Could you check a few things on this model? Use its own coordinates, in mm. A direction names the side the tool comes from. Coordinates: 2 decimals unless noted, no trailing zeros. Loops run counter-clockwise (first coordinate to the right, second up) from the corner with the lowest first, then second, coordinate; pieces in that order, holes last. Notation, with made-up numbers: (-21.75, 35) -> (23.25, 35) arc R10 cw to (23.25, 42) -> close; hole circle Ø3 at (-14, 36.25). An arc over 180 degrees is marked (long way). One line per question, with ' | ' between items.
from build123d import *
from OCP.BRepFilletAPI import BRepFilletAPI_MakeChamfer
from build123d.topology import SkipClean

# Parameters (mm, degrees)
SZKIC2_R                         = 1.25
DODANIE_WYCI_GNI_CIE2_DEPTH      = 2
DODANIE_WYCI_GNI_CIE3_DEPTH      = 3
DODANIE_WYCI_GNI_CIE3_DEPTH_BACK = 2
SZKIC3_W                         = 6
SZKIC3_H                         = 30
DODANIE_WYCI_GNI_CIE4_DEPTH      = 30
DODANIE_WYCI_GNI_CIE4_DEPTH_BACK = 2
SZKIC4_W                         = 6
SZKIC4_H                         = 3
SFAZOWANIE1_SIZE                 = 8
SFAZOWANIE1_SIZE2                = 7.929766182
SFAZOWANIE1_SIZE2_2              = 8.072133677
SFAZOWANIE2_SIZE                 = 10
SFAZOWANIE3_SIZE                 = 3
SZKIC5_W                         = 38.5
SZKIC5_H                         = 53.3
SZKIC5_W_2                       = 38.438336307
SZKIC5_H_2                       = 53.191798748
WYTNIJ_WYCI_GNI_CIE1_DEPTH       = 48.5
DODANIE_WYCI_GNI_CIE5_DEPTH      = 42.061663693
WYTNIJ_WYCI_GNI_CIE2_DEPTH       = 50.5


with BuildPart() as part:
    # Szkic2 → Dodanie-wyciągnięcie2 (new body)
    with BuildSketch(Plane.XY):
        with BuildLine():
            Line((-191.460111356, 62.995312244), (-303.460111356, 62.995312244))
            Line((-303.460111356, 62.995312244), (-308.460111356, 57.995312244))
            Line((-308.460111356, 57.995312244), (-308.460111356, 23.495312244))
            Line((-308.460111356, 23.495312244), (-303.460111356, 18.495312244))
            Line((-303.460111356, 18.495312244), (-302.736783969, 18.495312244))
            ThreePointArc((-302.736783969, 18.495312244), (-304.359873615, 24.570533036), (-302.660111356, 30.624749412))
            Line((-302.660111356, 30.624749412), (-302.660111356, 55.958269629))
            ThreePointArc((-302.660111356, 55.958269629), (-301.800506396, 56.364057485), (-301.339420723, 57.195312244))
            Line((-301.339420723, 57.195312244), (-283.580801989, 57.195312244))
            ThreePointArc((-283.580801989, 57.195312244), (-283.119716316, 56.364057485), (-282.260111356, 55.958269629))
            Line((-282.260111356, 55.958269629), (-282.260111356, 30.624749412))
            ThreePointArc((-282.260111356, 30.624749412), (-280.560349096, 24.570533036), (-282.183438743, 18.495312244))
            Line((-282.183438743, 18.495312244), (-257.736783969, 18.495312244))
            ThreePointArc((-257.736783969, 18.495312244), (-259.359873615, 24.570533036), (-257.660111356, 30.624749412))
            Line((-257.660111356, 30.624749412), (-257.660111356, 55.958269629))
            ThreePointArc((-257.660111356, 55.958269629), (-256.800506396, 56.364057485), (-256.339420723, 57.195312244))
            Line((-256.339420723, 57.195312244), (-238.580801989, 57.195312244))
            ThreePointArc((-238.580801989, 57.195312244), (-238.119716316, 56.364057485), (-237.260111356, 55.958269629))
            Line((-237.260111356, 55.958269629), (-237.260111356, 30.624749412))
            ThreePointArc((-237.260111356, 30.624749412), (-235.561787998, 24.695065265), (-237.060111356, 18.711714747))
            Line((-237.060111356, 18.711714747), (-212.736783969, 18.495312244))
            ThreePointArc((-212.736783969, 18.495312244), (-214.359873615, 24.570533036), (-212.660111356, 30.624749412))
            Line((-212.660111356, 30.624749412), (-212.660111356, 55.958269629))
            ThreePointArc((-212.660111356, 55.958269629), (-211.800506396, 56.364057485), (-211.339420723, 57.195312244))
            Line((-211.339420723, 57.195312244), (-193.580801989, 57.195312244))
            ThreePointArc((-193.580801989, 57.195312244), (-193.119716316, 56.364057485), (-192.260111356, 55.958269629))
            Line((-192.260111356, 55.958269629), (-192.260111356, 30.624749412))
            ThreePointArc((-192.260111356, 30.624749412), (-190.560349096, 24.570533036), (-192.183438743, 18.495312244))
            Line((-192.183438743, 18.495312244), (-191.460111356, 18.495312244))
            Line((-191.460111356, 18.495312244), (-186.460111356, 23.495312244))
            Line((-186.460111356, 23.495312244), (-186.460111356, 57.995312244))
            Line((-186.460111356, 57.995312244), (-191.460111356, 62.995312244))
        make_face()
        with Locations((-305.960111356, 31.245312244)):
            Circle(SZKIC2_R, mode=Mode.SUBTRACT)
        with Locations((-278.960111356, 31.245312244)):
            Circle(SZKIC2_R, mode=Mode.SUBTRACT)
        with Locations((-305.960111356, 39.245312244)):
            Circle(SZKIC2_R, mode=Mode.SUBTRACT)
        with Locations((-278.960111356, 39.245312244)):
            Circle(SZKIC2_R, mode=Mode.SUBTRACT)
        with Locations((-260.960111356, 31.245312244)):
            Circle(SZKIC2_R, mode=Mode.SUBTRACT)
        with Locations((-260.960111356, 39.245312244)):
            Circle(SZKIC2_R, mode=Mode.SUBTRACT)
        with Locations((-233.960111356, 31.245312244)):
            Circle(SZKIC2_R, mode=Mode.SUBTRACT)
        with Locations((-233.960111356, 39.245312244)):
            Circle(SZKIC2_R, mode=Mode.SUBTRACT)
        with Locations((-215.960111356, 31.245312244)):
            Circle(SZKIC2_R, mode=Mode.SUBTRACT)
        with Locations((-188.960111356, 31.245312244)):
            Circle(SZKIC2_R, mode=Mode.SUBTRACT)
        with Locations((-215.960111356, 39.245312244)):
            Circle(SZKIC2_R, mode=Mode.SUBTRACT)
        with Locations((-188.960111356, 39.245312244)):
            Circle(SZKIC2_R, mode=Mode.SUBTRACT)
        with Locations((-305.960111356, 47.245312244)):
            Circle(SZKIC2_R, mode=Mode.SUBTRACT)
        with Locations((-278.960111356, 47.245312244)):
            Circle(SZKIC2_R, mode=Mode.SUBTRACT)
        with Locations((-260.960111356, 47.245312244)):
            Circle(SZKIC2_R, mode=Mode.SUBTRACT)
        with Locations((-305.960111356, 55.245312244)):
            Circle(SZKIC2_R, mode=Mode.SUBTRACT)
        with Locations((-278.960111356, 55.245312244)):
            Circle(SZKIC2_R, mode=Mode.SUBTRACT)
        with Locations((-300.460111356, 60.495312244)):
            Circle(SZKIC2_R, mode=Mode.SUBTRACT)
        with Locations((-284.460111356, 60.495312244)):
            Circle(SZKIC2_R, mode=Mode.SUBTRACT)
        with Locations((-260.960111356, 55.245312244)):
            Circle(SZKIC2_R, mode=Mode.SUBTRACT)
        with Locations((-255.460111356, 60.495312244)):
            Circle(SZKIC2_R, mode=Mode.SUBTRACT)
        with Locations((-233.960111356, 47.245312244)):
            Circle(SZKIC2_R, mode=Mode.SUBTRACT)
        with Locations((-215.960111356, 47.245312244)):
            Circle(SZKIC2_R, mode=Mode.SUBTRACT)
        with Locations((-188.960111356, 47.245312244)):
            Circle(SZKIC2_R, mode=Mode.SUBTRACT)
        with Locations((-233.960111356, 55.245312244)):
            Circle(SZKIC2_R, mode=Mode.SUBTRACT)
        with Locations((-239.460111356, 60.495312244)):
            Circle(SZKIC2_R, mode=Mode.SUBTRACT)
        with Locations((-215.960111356, 55.245312244)):
            Circle(SZKIC2_R, mode=Mode.SUBTRACT)
        with Locations((-188.960111356, 55.245312244)):
            Circle(SZKIC2_R, mode=Mode.SUBTRACT)
        with Locations((-210.460111356, 60.495312244)):
            Circle(SZKIC2_R, mode=Mode.SUBTRACT)
        with Locations((-194.460111356, 60.495312244)):
            Circle(SZKIC2_R, mode=Mode.SUBTRACT)
    extrude(amount=DODANIE_WYCI_GNI_CIE2_DEPTH)

    # Szkic3 → Dodanie-wyciągnięcie3 (add, two sides: drawn at the far end of the back side and taken through both)
    with BuildSketch(Plane.XY.offset(2).offset(-DODANIE_WYCI_GNI_CIE3_DEPTH_BACK)):
        with Locations((-269.960111356, 27.695312244)):
            Rectangle(SZKIC3_W, SZKIC3_H)
        with Locations((-224.898447663, 27.803513496)):
            Rectangle(SZKIC3_W, SZKIC3_H)
    extrude(amount=DODANIE_WYCI_GNI_CIE3_DEPTH + DODANIE_WYCI_GNI_CIE3_DEPTH_BACK)

    # Szkic4 → Dodanie-wyciągnięcie4 (add, two sides: drawn at the far end of the back side and taken through both)
    with BuildSketch(Plane.XY.offset(2).offset(-DODANIE_WYCI_GNI_CIE4_DEPTH_BACK)):
        with Locations((-269.960111356, 11.195312244)):
            Rectangle(SZKIC4_W, SZKIC4_H)
        with Locations((-224.898447663, 11.303513496)):
            Rectangle(SZKIC4_W, SZKIC4_H)
    extrude(amount=DODANIE_WYCI_GNI_CIE4_DEPTH + DODANIE_WYCI_GNI_CIE4_DEPTH_BACK)

    # Sfazowanie1: one chamfer whose edges measure the first distance from different faces: ONE call of the kernel's chamfer builder (chamfer() names one face for all edges)
    sfazowanie1_edges_1 = [part.edges().sort_by_distance(p)[0] for p in [
        (-266.960111356, 18.495312244, 1),
        (-272.960111356, 18.495312244, 1),
    ]]
    sfazowanie1_edges_2 = [part.edges().sort_by_distance(p)[0] for p in [
        (-221.898447663, 18.57682276, 1),
    ]]
    sfazowanie1_side_2 = [part.faces().sort_by_distance(p)[0] for p in [
        (-221.898447663, 14.190168128, 0.459673797),
    ]]
    sfazowanie1_edges_3 = [part.edges().sort_by_distance(p)[0] for p in [
        (-227.898447663, 18.630204232, 1),
    ]]
    sfazowanie1_side_3 = [part.faces().sort_by_distance(p)[0] for p in [
        (-227.898447663, 42.343839698, 3.5),
    ]]
    sfazowanie1 = BRepFilletAPI_MakeChamfer(part.part.solid().wrapped)
    for e in sfazowanie1_edges_1:
        sfazowanie1.Add(SFAZOWANIE1_SIZE, e.wrapped)
    for e in sfazowanie1_edges_2:
        sfazowanie1.Add(SFAZOWANIE1_SIZE, SFAZOWANIE1_SIZE2, e.wrapped, sfazowanie1_side_2[0].wrapped)  # the first distance lies on this face
    for e in sfazowanie1_edges_3:
        sfazowanie1.Add(SFAZOWANIE1_SIZE, SFAZOWANIE1_SIZE2_2, e.wrapped, sfazowanie1_side_3[0].wrapped)  # the first distance lies on this face
    add(Compound.cast(sfazowanie1.Shape()), mode=Mode.REPLACE)

    # Sfazowanie2
    sfazowanie2_edges = [part.edges().sort_by_distance(p)[0] for p in [
        (-269.960111356, 12.695312244, 5),
        (-224.898447663, 12.803513496, 5),
    ]]
    chamfer(sfazowanie2_edges, length=SFAZOWANIE2_SIZE)

    # Sfazowanie3
    sfazowanie3_edges = [part.edges().sort_by_distance(p)[0] for p in [
        (-224.898447663, 12.803513496, 32),
        (-269.960111356, 12.695312244, 32),
        (-224.898447663, 42.803513496, 5),
        (-269.960111356, 42.695312244, 5),
    ]]
    chamfer(sfazowanie3_edges, length=SFAZOWANIE3_SIZE - 0.0001)  # a hair under: the kernel refuses the full size

    # Szkic5 → Wytnij-wyciągnięcie1 (cut, symmetric)
    with BuildSketch(Plane.XY.offset(2)):
        with Locations((-289.210111356, 36.345312244)):
            Rectangle(SZKIC5_W, SZKIC5_H)
        with Locations((-205.67927951, 36.39941287)):
            Rectangle(SZKIC5_W_2, SZKIC5_H_2)
    extrude(amount=WYTNIJ_WYCI_GNI_CIE1_DEPTH, both=True, mode=Mode.SUBTRACT)

    # Szkic6 → Dodanie-wyciągnięcie5 (add)
    with SkipClean():  # the faces are left unmerged after this step: merging them gives an invalid solid
        with BuildSketch(Plane(origin=(-266.960111356, 0, 0), x_dir=(0, 0, -1), z_dir=(1, 0, 0))):
            Polygon((-32, 9.695312244), (-29, 12.695312244), (0, 12.695312244), (0, 9.695312244), align=None)
        extrude(amount=DODANIE_WYCI_GNI_CIE5_DEPTH)

    # Szkic7 → Wytnij-wyciągnięcie2 (cut, symmetric)
    with BuildSketch(Plane.ZY.offset(269.960111356)):
        Polygon((5, 22.695312244), (5, 31.42772167), (32, 31.42772167), (32, 9.664251066), (29, 12.695312244), (15, 12.695312244), align=None)
    extrude(amount=WYTNIJ_WYCI_GNI_CIE2_DEPTH, both=True, mode=Mode.SUBTRACT)


solid = part.part
1) If we section it at C-C on z = 3.5: Please give me the cut outline in (x, y).
Data:
outline: (-269.96, 9.7) -> (-224.9, 9.7) -> (-224.9, 41.3) -> (-227.9, 41.3) -> (-227.9, 12.7) -> (-266.96, 12.7) -> (-266.96, 41.2) -> (-269.96, 41.2) -> close
2) I need wall thicknesses on line 1 along Y through (x, z) = (-244, 12); line 2 along Z through (x, y) = (-227, 48.5); line 3 along Z through (x, y) = (-227, 32). Which ranges of each line are inside material? Lowest first, please. Write a range as from..to.
Data:
line 1: 9.7..12.7 | line 2: 0..2 | line 3: 0..5
3) On a 3-axis mill with a long thin cutter (end or side, diameter ignored), from which of +Z, -Z, +X, -X, +Y, -Y can I reach the whole of each face in a straight line? I mean faces 4 (the face through (-227.898, 23, 4)), 5 (the face through (-258, 18.495, 1)), 6 (the face through (-268.481, 41.216, 3.479)). Say none if no direction works.
Data:
face 4: +Z, +Y | face 5: +Z, -Z | face 6: +Z, -X, +Y
4) We'd pull the mould along Y, two halves only. Please class faces 1 (the face through (-268, 31, 5)), 2 (the face through (-247.74, 11.17, 30.51)), 3 (the face through (-235.21, 55.3, 0.99)): pulls with the +Y half, pulls with the -Y half, needs draft (parallel to the pull), parting line crosses it, or undercut.
Data:
face 1: needs draft | face 2: pulls with the +Y half | face 3: undercut
5) I'm going to push flat-ended pins straight in: pin 1 Ø1.5 at (x, y) = (-233.96, 47.25) entering from -Z; pin 2 Ø8 at (x, z) = (-231.5, 21) entering from +Y; pin 3 Ø3 at (x, y) = (-239.46, 60.5) entering from +Z; pin 4 Ø3 at (x, y) = (-233.96, 55.25) entering from -Z. Where does each tip first touch, or does it pass through?
Data:
pin 1: through | pin 2: y = 12.7 | pin 3: z = 2 | pin 4: z = 0
6) If we section it at B-B on x = -252: Please give me the cut outline in (y, z).
Data:
outline: (9.7, 0) -> (12.7, 0) -> (12.7, 29) -> (9.7, 31.97) -> close; (57.2, 0) -> (63, 0) -> (63, 2) -> (57.2, 2) -> close
7) If we section it at D-D on y = 17: Please give me the cut outline in (x, z).
Data:
outline: (-269.96, 0) -> (-260.46, 0) -> (-260.46, 2) -> (-266.96, 2) -> (-266.96, 10.7) -> (-269.96, 10.7) -> close; (-234.27, 0) -> (-224.9, 0) -> (-224.9, 10.7) -> (-227.9, 10.7) -> (-227.9, 2) -> (-234.27, 2) -> close
8) If we section it at A-A on y = 44: Please give me the cut outline in (x, z), and give its area (3 significant figures).
Data:
outline: (-269.96, 0) -> (-257.66, 0) -> (-257.66, 2) -> (-269.96, 2) -> close; (-237.26, 0) -> (-224.9, 0) -> (-224.9, 2) -> (-237.26, 2) -> close | area: 49.3 mm²
